from build123d import *

# Parameters (mm, degrees)
F1_DEPTH = 63.5
F0_W     = 25.4
F0_H     = 19.0500000358
F2_DEPTH = 25.4
F4_DEPTH = 7.9375
F5_R     = 6.35


with BuildPart() as f1:
    # F0 (on Front) → F1 (new body, symmetric)
    with BuildSketch(Plane.XZ):
        Polygon((22.2249999642, 9.525), (-41.275, 9.525), (-41.275, -9.525), (41.275, -9.525), (41.275, 9.525), align=None)
    extrude(amount=F1_DEPTH, both=True)

    # F0 (on Front) → F2 (join, symmetric)
    with BuildSketch(Plane.XZ):
        with BuildLine():
            Line((22.2249999642, 22.8510349691), (22.2249999642, 9.525))
            Line((22.2249999642, 9.525), (41.275, 9.525))
            Line((41.275, 9.525), (41.275, 22.8510349691))
            ThreePointArc((41.275, 22.8510349691), (45.9246798487, 34.0763551205), (57.15, 38.7260349691))
            Line((57.15, 38.7260349691), (60.325, 38.7260349691))
            Line((60.325, 38.7260349691), (60.325, 57.7760350049))
            Line((60.325, 57.7760350049), (57.15, 57.7760350049))
            add(Edge.make_bspline(
                [(54.8082230388, 57.6974366221), (55.5907182934, 57.7282388811), (56.3713995227, 57.7544053824), (57.15, 57.7760350049)],
                knots=[107.3950550145, 107.3950550145, 107.3950550145, 107.3950550145, 109.6158884653, 109.6158884653, 109.6158884653, 109.6158884653], degree=3))
            ThreePointArc((54.8082230388, 57.6974366221), (31.6397845173, 46.7044316564), (22.2249999642, 22.8510349691))
        make_face()
        with Locations((73.025, 48.251034987)):
            Rectangle(F0_W, F0_H)
    extrude(amount=F2_DEPTH, both=True)

    # F0 (on Front) → F3 (revolve)
    with BuildSketch(Plane.XZ):
        Polygon((85.725, 66.675), (85.725, 57.7760350049), (85.725, 38.7260349691), (85.725, 34.925), (111.125, 34.925), (111.125, 66.675), align=None)
    revolve(axis=Axis((85.725, 0, 50.8), (0, 0, -1)))

    # F0 (on Front) → F4 (join, symmetric)
    with BuildSketch(Plane.XZ):
        with BuildLine():
            add(Edge.make_bspline(
                [(-41.275, 9.525), (-25.1136724024, 43.8776656842), (16.9683206865, 56.2079011061), (54.8082230388, 57.6974366221)],
                knots=[0, 0, 0, 0, 107.3950550145, 107.3950550145, 107.3950550145, 107.3950550145], degree=3))
            Line((-41.275, 9.525), (22.2249999642, 9.525))
            Line((22.2249999642, 9.525), (22.2249999642, 22.8510349691))
            ThreePointArc((22.2249999642, 22.8510349691), (31.6397845173, 46.7044316564), (54.8082230388, 57.6974366221))
        make_face()
    extrude(amount=F4_DEPTH, both=True)

    # F5
    f5_edges = [f1.edges().sort_by_distance(p)[0] for p in [
        (41.275, 63.5, 0),
        (-41.275, 63.5, 0),
        (41.275, -63.5, 0),
        (-41.275, -63.5, 0),
    ]]
    fillet(f5_edges, radius=F5_R)


solid = f1.part
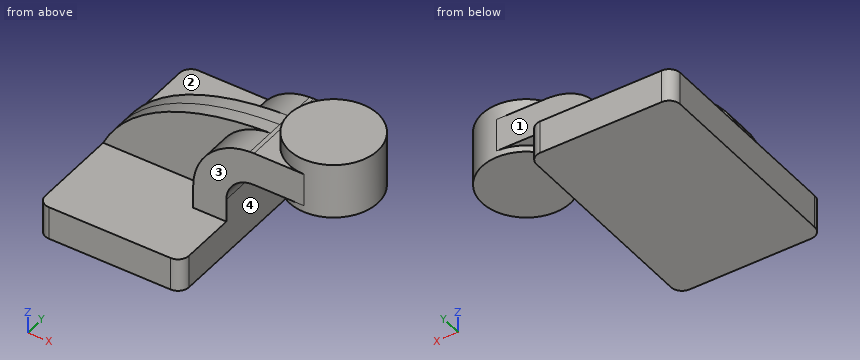
Check sheet for the modelled part. Datum: model origin and axes. Units: mm. Face numbers are marked on the shaded views. A direction names the side the tool comes from. Give positions to 0.01 mm unless a question says otherwise; leave off trailing zeros. Loops run counter-clockwise (first coordinate to the right, second up) from the corner with the lowest first, then second, coordinate; pieces in that order, holes last. Notation, with made-up numbers: M 71.5,28.5 L 79.5,28.5 A31 cw 79.5,54.5 Z; hole C -3.75,7.25 d7. An arc over 180 degrees is marked long. Answer as a JSON object with one key per item and string values. Group by question number.
Q1. Access from +Z, -Z, +X, -X, +Y, -Y to the whole of each face (thin tool, end or side, straight path). Record for the marked faces 1, 2, 3 and 4.
Q2. Cross-section at C-C on y = 32. Record the cut outline in (x, z) (3 decimals), then the cut area to 3 significant figures.
Q3. Material ranges on line 1 along X through (y, z) = (-54, -0.5) (3 decimals); line 2 along Y through (x, z) = (34, 21); line 3 along Y through (x, z) = (-24.5, 28.5), recorded low to high. Write a range as [from, to].
Q4. Go/stop test with flat-tipped pins: P1, Ø16, axis at y = -4, z = 10.5, coming from the +X side (3 decimals); P2, Ø24, axis at x = -10.5, z = 36, coming from the -Y side; P3, Ø14.5, axis at x = 18, z = 43, coming from the +Y side. Record where each tip stops, or that it passes through.
Q5. Cross-section at A-A on z = 1.5. Record the cut outline in (x, y) (3 decimals).
Q6. Cross-section at B-B on x = 74. Record the cut outline in (y, z) (3 decimals), then the cut area to 3 significant figures.
Evaluation:
{
 "1": {"face 1": "+Z, +X, -X, +Y", "face 2": "+Z, -X, +Y", "face 3": "+Z, +X, -X, -Y", "face 4": "-Z, +X, +Y, -Y"},
 "2": {"outline": "M -41.275,-9.525 L 41.275,-9.525 L 41.275,9.525 L -41.275,9.525 Z", "area": "1,570 mm2"},
 "3": {"line 1": "x = [-41.275, 41.275]", "line 2": "y = [-25.4, 25.4]", "line 3": "y = [-7.94, 7.94]"},
 "4": {"P1": "stops at x = 41.275", "P2": "stops at y = -7.94", "P3": "stops at y = 7.94"},
 "5": {"outline": "M -41.275,-57.15 A6.35 ccw -34.925,-63.5 L 34.925,-63.5 A6.35 ccw 41.275,-57.15 L 41.275,57.15 A6.35 ccw 34.925,63.5 L -34.925,63.5 A6.35 ccw -41.275,57.15 Z"},
 "6": {"outline": "M -25.4,38.726 L -22.532,38.726 L -22.532,34.925 L 22.532,34.925 L 22.532,38.726 L 25.4,38.726 L 25.4,57.776 L 22.532,57.776 L 22.532,66.675 L -22.532,66.675 L -22.532,57.776 L -25.4,57.776 Z", "area": "1,540 mm2"}
}
